Autodesk Inventor part; units mm, degrees
ref_plane "YZ Plane" through (0, 0, 0) normal (1, 0, 0) x (0, 1, 0)
ref_plane "XZ Plane" through (0, 0, 0) normal (0, 1, 0) x (-1, 0, 0)
ref_plane "XY Plane" through (0, 0, 0) normal (0, 0, 1) x (1, 0, 0)
sketch "Sketch1" plane through (0, 0, 0) normal (0, 0, 1) x (1, 0, 0)
  line L0 (47.7, 10.1753) -> (55.7, 10.1753)
  line L1 (55.7, -6.2247) -> (47.7, -6.2247)
  line L2 (47.7, -33.2316) -> (55.7, -33.2316)
  line L3 (55.7, -33.2316) -> (55.7, -16.8316)
  line L4 (55.7, -16.8316) -> (47.7, -16.8316)
  line L5 (60.2, -37.7316) -> (47.7, -37.7316)
  line L6 (60.2, -37.7316) -> (60.2, 14.6753)
  line L7 (55.7, -6.2247) -> (55.7, 10.1753)
  line L8 (47.7, 14.6753) -> (57.2, 14.6753)
  line L9 (47.7, -33.2316) -> (47.7, -37.7316)
  line L10 (47.7, 14.6753) -> (47.7, 10.1753)
  line L11 (47.7, -6.2247) -> (47.7, -16.8316)
  line L12 (60.2, 14.6753) -> (60.2, 29.6753)
  line L13 (60.2, 29.6753) -> (57.2, 29.6753)
  line L14 (57.2, 29.6753) -> (57.2, 14.6753)
extrude "Extrusion1" add sketch "Sketch1" along normal blind 18
sketch "Sketch2" plane through (0, 0, 18) normal (0, 0, 1) x (1, 0, 0)
  line L0 (60.2, 29.6753) -> (60.2, -37.7316) construction
  line L1 (47.7, -37.7316) -> (47.7, -33.2316) construction
  line L2 (60.2, -16.8316) -> (47.7, -16.8316)
  line L3 (47.7, -16.8316) -> (47.7, -37.7316)
  line L4 (47.7, -37.7316) -> (60.2, -37.7316)
  line L5 (60.2, -37.7316) -> (60.2, -16.8316)
  point P0 (0, 0)
extrude "Extrusion2" cut sketch "Sketch2" against normal blind 18
sketch "Sketch3" plane through (47.7, 14.6753, 0) normal (0, 1, 0) x (1, 0, 0)
  circle A0 centre (4, -4.5) radius 1.5
  circle A1 centre (4, -13.5) radius 1.5
  point P0 (-47.7, 0)
extrude "Extrusion3" cut sketch "Sketch3" against normal blind 4.5
sketch "Sketch4" plane through (47.7, -16.8316, 0) normal (-1, 0, 0) x (0, 0, 1)
  line L0 (0, 0) -> (18, 0) construction
  line L1 (15, 7.6069) -> (15, 0)
  line L2 (3, 0) -> (3, 7.6069)
  line L3 (3, 7.6069) -> (15, 7.6069)
  line L4 (3, 0) -> (15, 0)
  point P0 (0, 16.8316)
extrude "Extrusion4" cut sketch "Sketch4" against normal blind 20
sketch "Sketch5" plane through (55.7, -6.2247, 0) normal (-1, 0, 0) x (0, 0, 1)
  line L0 (0, 0) -> (0, 16.4) construction
  line L1 (0, 0) -> (18, 0) construction
  line L2 (18, 16.4) -> (18, 0) construction
  line L3 (0, 16.4) -> (18, 16.4) construction
  line L4 (3, 13.4) -> (3, 3)
  line L5 (3, 3) -> (15, 3)
  line L6 (15, 3) -> (15, 13.4)
  line L7 (15, 13.4) -> (3, 13.4)
  point P0 (0, 6.2247)
  dimension "d17" = 3
extrude "Extrusion5" cut sketch "Sketch5" against normal up to next
properties part number "pixyCam_mount"
Geometry: final body of the model. Coordinates: model frame, mm. A direction names the side the tool comes from. Round coordinates to 2 decimals unless told otherwise and drop trailing zeros. Loops run counter-clockwise (first coordinate to the right, second up) from the corner with the lowest first, then second, coordinate; pieces in that order, holes last.
Q1. Access query for faces 1 (the flat face through (54, -16.832, 2)), 2 (the flat face through (58, 2, 15)), 3 (the cylindrical face through (50.5, 12.5, 14.4)), 4 (the flat face through (55.7, 7.33, 8.87)), 5 (the flat face through (54, -13, 15)). Directions: +Z, -Z, +X, -X, +Y, -Y. A direction counts if a zero-diameter tool reaches every point of the face in a straight line with its end or side. Return the directions, or none.
Q2. Section C-C on x = 59.5. Return loops of the section in (y, z).
Q3. Section B-B on y = -13. Return loops of the section in (x, z), plus the area to 3 significant figures.
Q4. Material intervals for L1, parallel to Z at x = 51.7, y = 13.15; L2, parallel to Y at x = 54.5, z = 14.25; L3, parallel to Y at x = 55, z = 1.5, sorted ascending.
Q5. Pull-direction query (Y, two-part tool) for faces 6 (the flat face through (57.2, 22, 9)), 7 (the flat face through (58, 2, 3)), 8 (the flat face through (52, 14.675, 9)), 9 (the flat face through (52, 10.175, 9)); classes: released by +Y, released by -Y, zero draft, split by the parting line, or undercut.
Q6. Section A-A on z = 4.5. Return loops of the section in (x, y).
Q7. Pin query (flat end, axial travel): P1, Ø2.5, axis at x = 53.5, z = 9.5, coming from the -Y side; P2, Ø4, axis at x = 51.7, z = 4.5, coming from the +Y side; P3, Ø2.5, axis at x = 51.7, z = 13.5, coming from the +Y side. Return the tip coordinate at first contact, or that it passes through.
Q8. Section D-D on z = 7.5. Return loops of the section in (x, y).
Evaluation:
1. face 1: +Z, -Z, +X, -X, -Y
1. face 2: +X, -X
1. face 3: +Y
1. face 4: +Z, -Z, -X
1. face 5: +X, -X, -Y
2. outline: (-16.83, 0) - (29.68, 0) - (29.68, 18) - (-16.83, 18) - (-16.83, 15) - (-9.22, 15) - (-9.22, 3) - (-16.83, 3) - close; hole (-3.22, 3) - (7.18, 3) - (7.18, 15) - (-3.22, 15) - close
3. outline: (47.7, 0) - (60.2, 0) - (60.2, 3) - (47.7, 3) - close; (47.7, 15) - (60.2, 15) - (60.2, 18) - (47.7, 18) - close
3. area: 75.0 mm2
4. L1: z = 0 to 3, 6 to 12, 15 to 18
4. L2: y = -9.22 to -6.22, 10.18 to 14.68
4. L3: y = -16.83 to -6.22, 10.18 to 14.68
5. face 6: zero draft
5. face 7: undercut
5. face 8: released by +Y
5. face 9: undercut
6. outline: (47.7, -9.22) - (60.2, -9.22) - (60.2, -3.22) - (55.7, -3.22) - (55.7, -6.22) - (47.7, -6.22) - close; (47.7, 10.18) - (50.2, 10.18) - (50.2, 14.68) - (47.7, 14.68) - close; (53.2, 10.18) - (55.7, 10.18) - (55.7, 7.18) - (60.2, 7.18) - (60.2, 29.68) - (57.2, 29.68) - (57.2, 14.68) - (53.2, 14.68) - close
7. P1: stops at y = -9.22
7. P2: stops at y = 14.68
7. P3: stops at y = -6.22
8. outline: (47.7, -9.22) - (60.2, -9.22) - (60.2, -3.22) - (55.7, -3.22) - (55.7, -6.22) - (47.7, -6.22) - close; (47.7, 10.18) - (55.7, 10.18) - (55.7, 7.18) - (60.2, 7.18) - (60.2, 29.68) - (57.2, 29.68) - (57.2, 14.68) - (47.7, 14.68) - close
